The listing builds one solid part. Answer for the finished solid, in the listing's coordinates (mm). A direction names the side the tool comes from. Round coordinates to 2 decimals unless told otherwise and drop trailing zeros. Write each loop counter-clockwise with the first axis right and the second up, starting at its lowest first coordinate (ties: lowest second). Pieces come first, ordered by that corner, then holes.
Item 1: Find the intervals of material crossed by probe 1 along Y at (x, z) = (54, -35); probe 2 along X at (y, z) = (103, -5); probe 3 along Z at (x, y) = (27.5, 34.5), in increasing order.
Item 2: Find section A-A on x = 44. Give the vertices of the cut face in (y, z), then the cut area to 3 significant figures.
Item 3: For a pull along Y with two mould halves and no side action, classify faces 1 (the face through (4, 109, 1)), 2 (the face through (-97.15, 46.99, 0.59)), 3 (the face through (-96.99, 19.72, -49.65)) as +Y half, -Y half, draft (parallel to the pull), parting line (faces both ways), or undercut.
Item 4: A tool of negligible diameter and unlimited length cuts with its end or side. For faces 4 (the face through (-83.78, -9.3, 1.08)), 5 (the face through (-79, -60, 0)), 6 (the face through (43, 109, 40)), from which of +Z, -Z, +X, -X, +Y, -Y can it reach the whole face along a straight path? Write none if from no direction.
Item 5: Each of these flat-tipped pins is pushed along its axis until it touches: pin 1 (3 mm diameter, centred on y = 28, z = -12.5, fed in from +X); pin 2 (2 mm diameter, centred on y = 5, z = -5.5, fed in from +X); pin 3 (2 mm diameter, centred on x = -39, z = -37.5, fed in from +Y). Where does it stop, or does it pass through?
```python
from build123d import *

# Parameters (mm, degrees)
SKETCH2_W               = 200
SKETCH2_H               = 105
SKETCH2_R               = 7.75
BOSS_EXTRUDE2_DEPTH     = 50
SKETCH3_R               = 15
CUT_EXTRUDE1_DEPTH      = 40
SKETCH4_R               = 5
BOSS_EXTRUDE3_DEPTH     = 100
SKETCH5_W               = 112
SKETCH5_H               = 105
BOSS_EXTRUDE4_DEPTH     = 180
SKETCH7_R               = 7.75
CUT_EXTRUDE2_DEPTH      = 200
CUT_EXTRUDE3_DEPTH      = 160
CUT_EXTRUDE3_DEPTH_BACK = 40
SKETCH8_W               = 80
SKETCH8_H               = 80
FILLET6_R               = 10
FILLET7_R               = 10
FILLET8_R               = 10
FILLET9_R               = 50
FILLET10_R              = 50
FILLET11_R              = 50
FILLET12_R              = 50
FILLET14_R              = 10


with BuildPart() as part:
    # Sketch2 → Boss-Extrude2 (new body)
    with BuildSketch(Plane(origin=(0, 0, 0), x_dir=(1, 0, 0), z_dir=(0, 1, 0))):
        Rectangle(SKETCH2_W, SKETCH2_H)
        with Locations(Location((44, 0, 0), (0, 0, 270))):
            Circle(SKETCH2_R, mode=Mode.SUBTRACT)
    extrude(amount=BOSS_EXTRUDE2_DEPTH)

    # Sketch3 → Cut-Extrude1 (cut)
    with BuildSketch(Plane.XZ):
        with Locations(Location((-78.898621146, 0, 0), (0, 0, 270))):
            Circle(SKETCH3_R)
    extrude(amount=-CUT_EXTRUDE1_DEPTH, mode=Mode.SUBTRACT)

    # Sketch4 → Boss-Extrude3 (add)
    with BuildSketch(Plane.XZ.offset(-40)):
        with Locations(Location((-78.898621146, 0, 0), (0, 0, 270))):
            Circle(SKETCH4_R)
    extrude(amount=BOSS_EXTRUDE3_DEPTH)

    # Sketch5 → Boss-Extrude4 (add)
    with BuildSketch(Plane(origin=(0, 50, 0), x_dir=(1, 0, 0), z_dir=(0, 1, 0))):
        with Locations((44, 0)):
            Rectangle(SKETCH5_W, SKETCH5_H)
    extrude(amount=BOSS_EXTRUDE4_DEPTH)

    # Sketch7 → Cut-Extrude2 (cut)
    with BuildSketch(Plane.XZ.offset(-50)):
        with Locations(Location((44, 0, 0), (0, 0, 90))):
            Circle(SKETCH7_R)
    extrude(amount=-CUT_EXTRUDE2_DEPTH, mode=Mode.SUBTRACT)

    # Sketch8 → Cut-Extrude3 (cut, two sides: drawn at the far end of the back side and taken through both)
    with BuildSketch(Plane(origin=(0, 50, 0), x_dir=(1, 0, 0), z_dir=(0, 1, 0)).offset(-CUT_EXTRUDE3_DEPTH_BACK)):
        with Locations((44, 0)):
            Rectangle(SKETCH8_W, SKETCH8_H)
    extrude(amount=CUT_EXTRUDE3_DEPTH + CUT_EXTRUDE3_DEPTH_BACK, mode=Mode.SUBTRACT)

    # Fillet6
    # the kernel refuses this fillet: 10 mm, written as the material it takes off along each edge
    with BuildSketch(Plane(origin=(-100, 50, 77.5), x_dir=(0, -1, 0), z_dir=(0, 0, -1))) as fillet6_piece_1:
        with BuildLine():
            CenterArc((FILLET6_R, -FILLET6_R), FILLET6_R, 90, 90)
            Line((0, -FILLET6_R), (0, 0))
            Line((0, 0), (FILLET6_R, 0))
        make_face()
    extrude(amount=155, mode=Mode.SUBTRACT)
    with BuildSketch(Plane(origin=(-100, 0, 77.5), x_dir=(0, 1, 0), z_dir=(0, 0, -1))) as fillet6_piece_2:
        with BuildLine():
            CenterArc((FILLET6_R, FILLET6_R), FILLET6_R, 180, 90)
            Line((0, FILLET6_R), (0, 0))
            Line((0, 0), (FILLET6_R, 0))
        make_face()
    extrude(amount=155, mode=Mode.SUBTRACT)
    with BuildSketch(Plane(origin=(-100, -25, 52.5), x_dir=(0, 0, -1), z_dir=(0, 1, 0)), Plane(origin=(-100, -25, -52.5), x_dir=(1, 0, 0), z_dir=(0, 1, 0))) as fillet6_piece_3:
        with BuildLine():
            CenterArc((FILLET6_R, -FILLET6_R), FILLET6_R, 90, 90)
            Line((0, -FILLET6_R), (0, 0))
            Line((0, 0), (FILLET6_R, 0))
        make_face()
    extrude(amount=100, mode=Mode.SUBTRACT)

    # Fillet7
    # the kernel refuses this fillet: 10 mm, written as the material it takes off along each edge
    with BuildSketch(Plane(origin=(-90, 40, 42.5), x_dir=(0, 0, 1), z_dir=(0, 1, 0))) as fillet7_piece_1_section:
        Polygon((0, 0), (FILLET7_R, 0), (FILLET7_R, -FILLET7_R), (0, -FILLET7_R), align=None)
    fillet7_piece_1 = extrude(amount=FILLET7_R, mode=Mode.PRIVATE)
    fillet7_piece_1 = fillet7_piece_1 - Plane(origin=(-90, 40, 42.5), x_dir=(0.7071067811865477, 0, -0.7071067811865475), z_dir=(0, 1, 0)) * Sphere(FILLET7_R, mode=Mode.PRIVATE)
    add(fillet7_piece_1, mode=Mode.SUBTRACT)
    with BuildSketch(Plane(origin=(-12, 50, 52.5), x_dir=(0, 0, -1), z_dir=(-1, 0, 0))) as fillet7_piece_2:
        with BuildLine():
            CenterArc((FILLET7_R, FILLET7_R), FILLET7_R, 180, 90)
            Line((0, FILLET7_R), (0, 0))
            Line((0, 0), (FILLET7_R, 0))
        make_face()
    extrude(amount=78, mode=Mode.SUBTRACT)

    # Fillet8
    # the kernel refuses this fillet: 10 mm, written as the material it takes off along each edge
    with BuildSketch(Plane(origin=(-90, 40, -42.5), x_dir=(0, 1, 0), z_dir=(0, 0, -1))) as fillet8_piece_1_section:
        Polygon((0, 0), (FILLET8_R, 0), (FILLET8_R, -FILLET8_R), (0, -FILLET8_R), align=None)
    fillet8_piece_1 = extrude(amount=FILLET8_R, mode=Mode.PRIVATE)
    fillet8_piece_1 = fillet8_piece_1 - Plane(origin=(-90, 40, -42.5), x_dir=(0.7071067811865475, -0.7071067811865475, 0), z_dir=(0, 0, -1)) * Sphere(FILLET8_R, mode=Mode.PRIVATE)
    add(fillet8_piece_1, mode=Mode.SUBTRACT)
    with BuildSketch(Plane(origin=(-90, 50, -52.5), x_dir=(0, -1, 0), z_dir=(1, 0, 0))) as fillet8_piece_2:
        with BuildLine():
            CenterArc((FILLET8_R, -FILLET8_R), FILLET8_R, 90, 90)
            Line((0, -FILLET8_R), (0, 0))
            Line((0, 0), (FILLET8_R, 0))
        make_face()
    extrude(amount=78, mode=Mode.SUBTRACT)

    # Fillet9
    fillet9_edges = [part.edges().sort_by_distance(p)[0] for p in [
        (100, 115, 52.5),
    ]]
    fillet(fillet9_edges, radius=FILLET9_R)

    # Fillet10
    fillet10_edges = [part.edges().sort_by_distance(p)[0] for p in [
        (-12, 135, 52.5),
    ]]
    fillet(fillet10_edges, radius=FILLET10_R)

    # Fillet11
    fillet11_edges = [part.edges().sort_by_distance(p)[0] for p in [
        (100, 115, -52.5),
    ]]
    fillet(fillet11_edges, radius=FILLET11_R)

    # Fillet12
    fillet12_edges = [part.edges().sort_by_distance(p)[0] for p in [
        (-12, 135, -52.5),
    ]]
    fillet(fillet12_edges, radius=FILLET12_R)

    # Fillet14
    fillet14_edges = [part.edges().sort_by_distance(p)[0] for p in [
        (100, 230, 0),
        (85.355339059, 230, 37.855339059),
        (44, 230, 52.5),
        (2.644660941, 230, 37.855339059),
        (44, 230, -52.5),
        (85.355339059, 230, -37.855339059),
        (-12, 230, 0),
        (2.644660941, 230, -37.855339059),
    ]]
    fillet(fillet14_edges, radius=FILLET14_R)


solid = part.part
```
Check values:
1. probe 1: y = 0 to 10, 210 to 230
1. probe 2: x = -11.94 to 4, 84 to 99.94
1. probe 3: z = -52.5 to -40, 40 to 52.5
2. outline: (0, -52.5) - (220, -52.5) arc R10 ccw to (230, -42.5) - (230, -7.75) - (210, -7.75) - (210, -40) - (10, -40) - (10, -7.75) - (0, -7.75) - close; (0, 7.75) - (10, 7.75) - (10, 40) - (210, 40) - (210, 7.75) - (230, 7.75) - (230, 42.5) arc R10 ccw to (220, 52.5) - (0, 52.5) - close
2. area: 7,640 mm2
3. face 1: undercut
3. face 2: +Y half
3. face 3: draft
4. face 4: -Y
4. face 5: +Z, -Z, +X, -X, -Y
4. face 6: none
5. pin 1: stops at x = 99.27
5. pin 2: stops at x = 99.96
5. pin 3: stops at y = 50
